Input: part model. Units: mm. Frame: model coordinates. Face numbers are marked on the shaded views. A direction names the side the tool comes from. Give positions to 0.01 mm unless a question says otherwise; leave off trailing zeros. Loops run counter-clockwise (first coordinate to the right, second up) from the corner with the lowest first, then second, coordinate; pieces in that order, holes last. Notation, with made-up numbers: M 8.5,-31 L 59.5,-31 A20 cw 59.5,-14 Z; hole C 35.5,55.5 d11. An arc over 180 degrees is marked long. One line per item, written item: value. Start each with the question number.
(1) Section A-A on x = 10.5. Output: boundary loops of the cut face in (y, z).
(2) Pull-direction query (X, two-part tool) for the marked faces 1, 2 and 3; classes: released by +X, released by -X, zero draft, split by the parting line, or undercut.
(3) Access query for the marked faces 4 and 5. Directions: +Z, -Z, +X, -X, +Y, -Y. A direction counts if a zero-diameter tool reaches every point of the face in a straight line with its end or side. Return the directions, or none.
(4) Section B-B on x = 1.5. Output: boundary loops of the cut face in (y, z).
(5) Pin query (flat end, axial travel): P1, Ø2, axis at x = 4, y = -2, coming from the -Z side; P2, Ø1, axis at x = 9.5, z = 0, coming from the +Y side; P3, Ø6, axis at x = 16, y = 3.5, coming from the -Z side. Return the tip coordinate at first contact, or that it passes through.
(6) Ray query, line 1 along X through (y, z) = (7.5, 0.5); line 2 along Z through (x, y) = (4, -3.25); line 3 along Z through (x, y) = (4.5, 5.25). Return the intervals inside material, ascending. Write a range as from..to.
```python
from build123d import *

# Parameters (mm, degrees)
CHAMFER1_SIZE = 0.35


with BuildPart() as part:
    # Sketch1 → Revolve1 (revolve)
    with BuildSketch(Plane.XY):
        Polygon((0, 0), (0, 8), (1, 8), (1, 6.8), (4.6, 6.8), (4.6, 5.6), (8.2, 5.6), (8.2, 4.4), (11.8, 4.4), (11.8, 3.2), (15.4, 3.2), (15.4, 2), (19, 2), (19, 3), (20, 3), (20, 0), align=None)
    revolve(axis=Axis((20, 0, 0), (-1, 0, 0)))

    # Chamfer1
    chamfer1_edges = [part.edges().sort_by_distance(p)[0] for p in [
        (15.4, -2, 0),
        (15.4, -3.2, 0),
        (11.8, -3.2, 0),
        (11.8, -4.4, 0),
        (8.2, -4.4, 0),
        (8.2, -5.6, 0),
        (4.6, -5.6, 0),
        (4.6, -6.8, 0),
    ]]
    chamfer(chamfer1_edges, length=CHAMFER1_SIZE)


solid = part.part
```
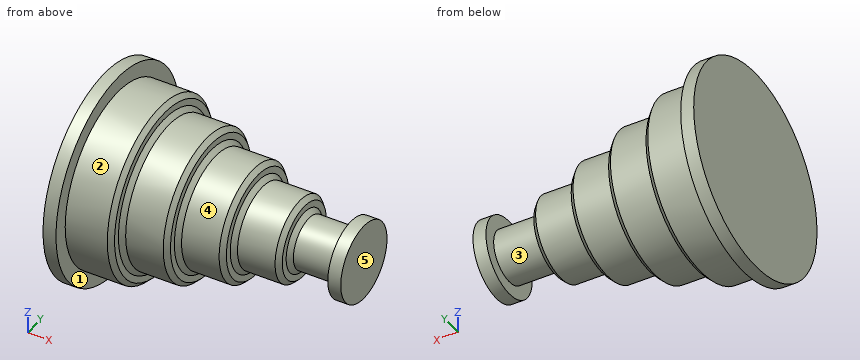
Output values:
1. outline: C 0,0 d8.8
2. face 1: released by +X
2. face 2: zero draft
2. face 3: undercut
3. face 4: +X
3. face 5: +Z, -Z, +X, +Y, -Y
4. outline: C 0,0 d13.6
5. P1: stops at z = -6.73
5. P2: stops at y = 4.4
5. P3: stops at z = -3.13
6. line 1: x = 0..1
6. line 2: z = -5.97..5.97
6. line 3: z = -3.92..3.92
